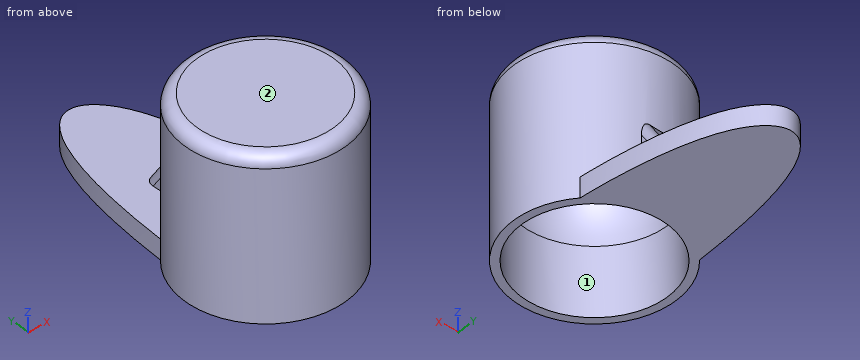
```python
from build123d import *

# Parameters (mm, degrees)
SKETCH_R     = 20
PAD_DEPTH    = 40
SKETCH001_R  = 18
POCKET_DEPTH = 35
FILLET_R     = 18
FILLET001_R  = 3
PAD001_DEPTH = 5
PAD002_DEPTH = 5
FILLET002_R  = 2


with BuildPart() as part:
    # Sketch → Pad (new body)
    with BuildSketch(Plane.XY):
        Circle(SKETCH_R)
    extrude(amount=PAD_DEPTH)

    # Sketch001 (on Face2 of Pad) → Pocket (cut)
    with BuildSketch(Plane(origin=(0, 0, 0), x_dir=(1, 0, 0), z_dir=(0, 0, -1))):
        Circle(SKETCH001_R)
    extrude(amount=-POCKET_DEPTH, mode=Mode.SUBTRACT)

    # Fillet
    fillet_edges = [part.edges().sort_by_distance(p)[0] for p in [
        (-18, 0, 35),
    ]]
    fillet(fillet_edges, radius=FILLET_R)

    # Fillet001
    fillet001_edges = [part.edges().sort_by_distance(p)[0] for p in [
        (-20, 0, 40),
    ]]
    fillet(fillet001_edges, radius=FILLET001_R)

    # Sketch002 (on Face3 of Fillet001) → Pad001 (join)
    with BuildSketch(Plane(origin=(0, 0, 0), x_dir=(1, 0, 0), z_dir=(0, 0, -1))):
        with BuildLine():
            add(Edge.make_bspline(
                [(-15, -13.228757), (-12.5, -60.801779), (12.5, -60.801779), (15, -13.228757), (15, -13.228757)],
                knots=[0, 0, 0, 0, 0.5, 1, 1, 1, 1], degree=3))
            Line((15, -13.228757), (9.755599, -16.368215))
            Line((9.755599, -16.368215), (2.922141, -18.626266))
            Line((2.922141, -18.626266), (-4.636806, -18.626266))
            Line((-4.636806, -18.626266), (-15, -13.228757))
        make_face()
    extrude(amount=-PAD001_DEPTH)

    # Sketch003 (on DatumPlane) → Pad002 (join, symmetric)
    with BuildSketch(Plane(origin=(-0.443704, 36.200309, 2.5), x_dir=(0, 0, -1), z_dir=(0.999439, 0.033491, 0))):
        Polygon((-2.4, -16.790791), (-17.4, -16.790791), (-2.4, -6.790791), align=None)
    extrude(amount=PAD002_DEPTH, both=True)

    # Fillet002
    fillet002_edges = [part.edges().sort_by_distance(p)[0] for p in [
        (-5.047294, 24.286952, 12.342556),
        (4.949495, 24.550274, 12.45),
    ]]
    fillet(fillet002_edges, radius=FILLET002_R)


solid = part.part
```
Design review of the part built by this model. Coordinates are the model's own, in mm. Face numbers are marked on the shaded views. Give positions to 0.01 mm unless a question says otherwise; leave off trailing zeros. Loops run counter-clockwise (first coordinate to the right, second up) from the corner with the lowest first, then second, coordinate; pieces in that order, holes last. Notation, with made-up numbers: M 72,-2 L 90,-2 A15 cw 90,22 Z; hole C 20.5,77 d3. An arc over 180 degrees is marked long. Return JSON: item names as keys, results as strings. Group by question number.
Item 1: Insertion check: pin 1 Ø10 at (x, y) = (4, 5.5) entering from -Z; pin 2 Ø9 at (x, y) = (6, 31) entering from +Z; pin 3 Ø10 at (x, y) = (15, 6.5) entering from -Z; pin 4 Ø3 at (y, z) = (8, 16.5) entering from +X. Each pin has a flat end and moves straight along its axis. Give the tip position at first contact, or say it passes through.
Item 2: We need section A-A (y = 0). Give the boundary of the cut face in (x, z), and give its area (3 significant figures).
Item 3: We need section C-C (z = 27). Give the boundary of the cut face in (x, y), and give its area (3 significant figures).
Item 4: For probe 1 along X at (y, z) = (0, 12); probe 2 along Z at (x, y) = (-10.5, -8); probe 3 along Y at (x, z) = (0, 12.75), list the stretches that pass through material, from the lowest coordinate up.
Item 5: Mouldability with a two-part tool opening along X and no side actions: class the marked faces 1 and 2 as released by +X, released by -X, zero draft, split by the parting line, or undercut.
Item 6: We need section B-B (z = 22). Give the boundary of the cut face in (x, y), and give its area (3 significant figures).
Output:
{
 "1": {"pin 1": "stops at z = 30.59", "pin 2": "stops at z = 8.19", "pin 3": "stops at z = 0", "pin 4": "stops at x = 18.91"},
 "2": {"outline": "M -20,0 L -18,0 L -18,17 A18 cw 18,17 L 18,0 L 20,0 L 20,37 A3 ccw 17,40 L -17,40 A3 ccw -20,37 Z", "area": "475 mm^2"},
 "3": {"outline": "C 0,0 d40; hole C 0,0 d29.93", "area": "553 mm^2"},
 "4": {"probe 1": "x = -20 to -18, 18 to 20", "probe 2": "z = 29.24 to 40", "probe 3": "y = -20 to -18, 18 to 24.18"},
 "5": {"face 1": "undercut", "face 2": "zero draft"},
 "6": {"outline": "C 0,0 d40; hole C 0,0 d34.58", "area": "317 mm^2"}
}
